Autodesk Inventor part; units mm, degrees
ref_plane "YZ Plane" through (0, 0, 0) normal (1, 0, 0) x (0, 1, 0)
ref_plane "XZ Plane" through (0, 0, 0) normal (0, 1, 0) x (-1, 0, 0)
ref_plane "XY Plane" through (0, 0, 0) normal (0, 0, 1) x (1, 0, 0)
sketch "Sketch1" plane through (0, 0, 0) normal (0, 1, 0) x (-1, 0, 0)
  line L0 (0, 2.5) -> (60, 2.5)
  line L1 (60, 2.5) -> (60, -27.5)
  line L2 (60, -27.5) -> (0, -27.5)
  line L3 (0, -27.5) -> (0, 2.5)
  dimension "d0" = 60
  dimension "d1" = 30
  dimension "d2" = 60
  dimension "d164" = 90
  dimension "d165" = 90
extrude "Extrusion1" add sketch "Sketch1" against normal blind 5 and the other way blind 12
sketch "Sketch2" plane through (0, 12, 0) normal (0, 1, 0) x (1, 0, 0)
  line L0 (-60, 27.5) -> (-60, -2.5)
  line L1 (0, 0) -> (0, 30)
  line L2 (0, 27.5) -> (-60, 27.5)
  line L3 (-60, -2.5) -> (0, -2.5)
  line L4 (-5, 0) -> (-5, 30)
  point P0 (-40, 7.5)
  point P1 (-20, 7.5)
  dimension "d44" = 10
  dimension "d45" = 20
  dimension "d46" = 20
  dimension "d47" = 10
  dimension "d67" = 15
sketch "Sketch3" plane through (0, 12, 0) normal (0, 1, 0) x (1, 0, 0)
  line L0 (0, 27.5) -> (-60, 27.5)
  line L1 (-60, -2.5) -> (-60, 27.5)
  point P0 (0, 0)
  point P1 (-50, 22.5)
  point P2 (-5, 30)
  point P3 (-25, 22.5)
  dimension "d56" = 5
  dimension "d57" = 10
  dimension "d58" = 25
  dimension "d59" = 5
sketch "Sketch16" plane through (-60, -5, 2.5) normal (0, 0, 1) x (1, 0, 0)
  line L0 (60, 17) -> (0, 17)
  line L1 (24.5, 16.25) -> (24.5, 14)
  line L2 (24.5, 14) -> (35.5, 14)
  line L3 (35.5, 14) -> (35.5, 16.25)
  line L4 (35.5, 17) -> (24.5, 17)
  line L5 (60, 0) -> (0, 0)
  line L6 (0, 17) -> (60, 17)
  line L7 (24.5, 16.25) -> (24.5, 17)
  line L8 (35.5, 17) -> (35.5, 16.25)
  point P0 (60, 5)
  point P1 (25.5, 17)
  point P2 (30, 17)
  point P3 (30, 0)
  point P4 (30, 17)
  point P5 (30, 0)
  point P6 (30, 17)
  point P7 (30, 0)
  dimension "d90" = 1
  dimension "d92" = 2.25
  dimension "d93" = 11
extrude "Extrusion6" cut sketch "Sketch16" against normal up to next
sketch "Sketch17" plane through (-35.5, 9, 2.5) normal (0, 1, 0) x (1, 0, 0)
  circle A0 centre (5.5, 8) radius 1.5
  line L0 (0, 30) -> (11, 30)
  line L1 (11, 0) -> (0, 0)
  point P0 (35.5, 2.5)
  point P1 (5.5, 30)
  dimension "d97" = 3
  dimension "d155" = 8
extrude "Extrusion7" cut sketch "Sketch17" against normal up to next
ref_plane "Work Plane2" through (0, 15.5, 0) normal (0, 1, 0) x (1, 0, 0)
sketch "Sketch21" plane through (0, -5, 0) normal (0, -1, 0) x (1, 0, 0)
  circle A0 centre (-12, -22) radius 4
  circle A1 centre (-48, -22) radius 4
  point P0 (0, 0)
  dimension "d125" = 8
  dimension "d131" = 8
extrude "Extrusion13" cut sketch "Sketch21" against normal blind 12
sketch "Sketch23" plane through (-12, 7, -22) normal (0, -1, 0) x (1, 0, 0)
  circle A0 centre (0, 0) radius 1.5
  circle A1 centre (-36, 0) radius 1.5
  point P0 (12, 22)
  dimension "d134" = 3
  dimension "d135" = 3
extrude "Extrusion14" cut sketch "Sketch23" against normal up to next
sketch "Sketch25" plane through (0, 12, 0) normal (0, 1, 0) x (1, 0, 0)
  circle A0 centre (-22, 5) radius 1.5
  circle A1 centre (-22, 20) radius 1.5
  circle A2 centre (-38, 20) radius 1.5
  circle A3 centre (-38, 5) radius 1.5
  line L0 (-60, -2.5) -> (0, -2.5)
  line L1 (-60, 27.5) -> (-60, -2.5)
  point P0 (0, 0)
  point P1 (-34.5, 0)
  dimension "d145" = 3
  dimension "d146" = 3
  dimension "d147" = 3
  dimension "d148" = 3
  dimension "d149" = 16
  dimension "d150" = 15
  dimension "d151" = 7.5
  dimension "d152" = 22
extrude "Extrusion16" cut sketch "Sketch25" against normal up to next
sketch "Sketch26" plane through (0, 12, 0) normal (0, 1, 0) x (1, 0, 0)
  circle A0 centre (-38, 20) radius 3
  circle A1 centre (-22, 20) radius 3
  circle A2 centre (-38, 5) radius 3
  circle A3 centre (-22, 5) radius 3
  line L0 (-60, -2.5) -> (-35.5, -2.5)
  point P0 (0, 0)
  dimension "d156" = 6
  dimension "d157" = 6
  dimension "d160" = 6
  dimension "d161" = 6
  dimension "d166" = 15
  dimension "d167" = 16
  dimension "d168" = 7.5
extrude "Extrusion18" cut sketch "Sketch26" against normal blind 8
sketch "Sketch11" plane through (0, 12, 0) normal (0, 1, 0) x (1, 0, 0)
  point P0 (-20, 10)
  point P1 (-40, 10)
properties part number "detalKKoretke"
Build history of the part. All positions in model axes, mm. A direction names the side the tool comes from. Round coordinates to 2 decimals unless told otherwise and drop trailing zeros. Loops run counter-clockwise (first coordinate to the right, second up) from the corner with the lowest first, then second, coordinate; pieces in that order, holes last. Notation, with made-up numbers: M -3.5,-3.75 L 30.5,-3.75 A31 cw 30.5,32.25 Z; hole C -21,50.5 d3. An arc over 180 degrees is marked long. Answer as CSV lines item,"result".
1. Flat gauge pins, fed straight in: P1, Ø6.5, axis at x = -12, z = -22, coming from the -Y side; P2, Ø3, axis at x = -38.5, z = -4, coming from the +Y side. Where does each tip first touch, or does it go through?
Resolved:
P1,"stops at y = 7"
P2,"stops at y = 4"
2. Cut at A-A on x = -22. Write the cut outline in (y, z), then the cut area to 3 significant figures.
Resolved:
outline,"M -5,-27.5 L 12,-27.5 L 12,-23 L 4,-23 L 4,-21.5 L -5,-21.5 Z; M -5,-18.5 L 4,-18.5 L 4,-17 L 12,-17 L 12,-8 L 4,-8 L 4,-6.5 L -5,-6.5 Z; M -5,-3.5 L 4,-3.5 L 4,-2 L 12,-2 L 12,2.5 L -5,2.5 Z"
area,"360 mm²"
3. Wall check: probe 1 along Z at (x, y) = (-22, 6.75); probe 2 along Z at (x, y) = (-22, -2); probe 3 along X at (y, z) = (1.5, -20). Give the ranges that are in metal, low to high. Write a range as [from, to].
Resolved:
probe 1,"z = [-27.5, -23], [-17, -8], [-2, 2.5]"
probe 2,"z = [-27.5, -21.5], [-18.5, -6.5], [-3.5, 2.5]"
probe 3,"x = [-60, -51.46], [-44.54, -39.5], [-36.5, -23.5], [-20.5, -15.46], [-8.54, 0]"
4. 3-axis set-ups, long thin cutter, end or side, ignore diameter. For faces 1 (the flat face through (-35.5, 11, -12)), 2 (the cylindrical face through (-50.95, 0.92, -19.3)), 3 (the flat face through (-20.7, 4, -18.7)): which of +Z, -Z, +X, -X, +Y, -Y reach the whole face in a straight line?
Resolved:
face 1,"+Z, -Z, +Y"
face 2,"-Y"
face 3,"+Y"
5. Cut at D-D on x = -48. Write the cut outline in (y, z), then the cut area to 3 significant figures.
Resolved:
outline,"M -5,-27.5 L 12,-27.5 L 12,-23.5 L 7,-23.5 L 7,-26 L -5,-26 Z; M -5,-18 L 7,-18 L 7,-20.5 L 12,-20.5 L 12,2.5 L -5,2.5 Z"
area,"399 mm²"
6. Cut at C-C on z = -9.5. Write the cut outline in (x, y).
Resolved:
outline,"M -60,-5 L 0,-5 L 0,12 L -24.5,12 L -24.5,9 L -35.5,9 L -35.5,12 L -60,12 Z"
7. Cut at B-B on x = -30. Write the cut outline in (y, z), then the cut area to 3 significant figures.
Resolved:
outline,"M -5,-27.5 L 9,-27.5 L 9,-7 L -5,-7 Z; M -5,-4 L 9,-4 L 9,2.5 L -5,2.5 Z"
area,"378 mm²"
8. Two-plate mould, pull along X, no slides. Class faces 4 (the flat face through (0, 4, -13)), 5 (the flat face through (-30, -5, -12)), 6 (the cylindrical face through (-19.23, 8.06, -18.85)): released by +X, released by -X, zero draft, split by the parting line, or undercut.
Resolved:
face 4,"released by +X"
face 5,"zero draft"
face 6,"undercut"
